from build123d import *

# Parameters (mm, degrees)
CYLINDER042_R          = 4
CYLINDER042_DEPTH      = 61
CYLINDER042_ROLL_ANGLE = 90
CYLINDER047_R          = 4
CYLINDER047_DEPTH      = 45
CYLINDER047_ROLL_ANGLE = 90
CYLINDER045_R          = 1.75
CYLINDER045_DEPTH      = 31
CYLINDER045_ROLL_ANGLE = 90
CYLINDER046_R          = 4
CYLINDER046_DEPTH      = 45
CYLINDER046_ROLL_ANGLE = 90
CYLINDER043_R          = 6
CYLINDER043_DEPTH      = 63
CYLINDER043_ROLL_ANGLE = 90
BOX038_W               = 8
BOX038_H               = 58
BOX038_DEPTH           = 11
CYLINDER044_R          = 1.75
CYLINDER044_DEPTH      = 23
CYLINDER044_ROLL_ANGLE = 90
BOX040_W               = 81
BOX040_H               = 81
BOX040_DEPTH           = 6
FILLET018008_R         = 5
BOX039_W               = 76
BOX039_H               = 76
BOX039_DEPTH           = 66
FILLET018007_R         = 3


with BuildPart() as cylinder064:
    # Cylinder042 → Cylinder042 (new body)
    with BuildSketch(Plane.XY):
        Circle(CYLINDER042_R)
    extrude(amount=CYLINDER042_DEPTH)


with BuildPart() as cylinder064_1:
    # Cylinder042 roll: moved
    add(cylinder064.part.rotate(Axis((0, 0, 0), (1, 0, 0)), CYLINDER042_ROLL_ANGLE))


with BuildPart() as cylinder064_2:
    # Cylinder042 placement: moved
    add(cylinder064_1.part.moved(Location((-5, 124, 89.6))))


with BuildPart() as cylinder069:
    # Cylinder047 → Cylinder047 (new body)
    with BuildSketch(Plane.XY):
        Circle(CYLINDER047_R)
    extrude(amount=CYLINDER047_DEPTH)


with BuildPart() as cylinder069_1:
    # Cylinder047 roll: moved
    add(cylinder069.part.rotate(Axis((0, 0, 0), (1, 0, 0)), CYLINDER047_ROLL_ANGLE))


with BuildPart() as cylinder069_2:
    # Cylinder047 placement: moved
    add(cylinder069_1.part.moved(Location((-8.5, 124, 71.5))))


with BuildPart() as cylinder067:
    # Cylinder045 → Cylinder045 (new body)
    with BuildSketch(Plane.XY):
        Circle(CYLINDER045_R)
    extrude(amount=CYLINDER045_DEPTH)


with BuildPart() as cylinder067_1:
    # Cylinder045 roll: moved
    add(cylinder067.part.rotate(Axis((0, 0, 0), (1, 0, 0)), CYLINDER045_ROLL_ANGLE))


with BuildPart() as cylinder067_2:
    # Cylinder045 placement: moved
    add(cylinder067_1.part.moved(Location((-8.5, 94, 71.5))))


with BuildPart() as cylinder068:
    # Cylinder046 → Cylinder046 (new body)
    with BuildSketch(Plane.XY):
        Circle(CYLINDER046_R)
    extrude(amount=CYLINDER046_DEPTH)


with BuildPart() as cylinder068_1:
    # Cylinder046 roll: moved
    add(cylinder068.part.rotate(Axis((0, 0, 0), (1, 0, 0)), CYLINDER046_ROLL_ANGLE))


with BuildPart() as cylinder068_2:
    # Cylinder046 placement: moved
    add(cylinder068_1.part.moved(Location((-8.5, -7, 71.5))))


with BuildPart() as cylinder065:
    # Cylinder043 → Cylinder043 (new body)
    with BuildSketch(Plane.XY):
        Circle(CYLINDER043_R)
    extrude(amount=CYLINDER043_DEPTH)


with BuildPart() as cylinder065_1:
    # Cylinder043 roll: moved
    add(cylinder065.part.rotate(Axis((0, 0, 0), (1, 0, 0)), CYLINDER043_ROLL_ANGLE))


with BuildPart() as cylinder065_2:
    # Cylinder043 placement: moved
    add(cylinder065_1.part.moved(Location((-3, 11, 83.5))))


with BuildPart() as cube037:
    # Box038 → Box038 (new body)
    with BuildSketch(Plane(origin=(-11.5, -52, 95), x_dir=(1, 0, 0), z_dir=(0, 0, 1))):
        with Locations((4, 29)):
            Rectangle(BOX038_W, BOX038_H)
    extrude(amount=BOX038_DEPTH)


with BuildPart() as cylinder066:
    # Cylinder044 → Cylinder044 (new body)
    with BuildSketch(Plane.XY):
        Circle(CYLINDER044_R)
    extrude(amount=CYLINDER044_DEPTH)


with BuildPart() as cylinder066_1:
    # Cylinder044 roll: moved
    add(cylinder066.part.rotate(Axis((0, 0, 0), (1, 0, 0)), CYLINDER044_ROLL_ANGLE))


with BuildPart() as cylinder066_2:
    # Cylinder044 placement: moved
    add(cylinder066_1.part.moved(Location((-8.5, 1, 71.5))))


with BuildPart() as fillet018008:
    # Box040 → Box040 (new body)
    with BuildSketch(Plane(origin=(-23.5, -4.5, 63), x_dir=(1, 0, 0), z_dir=(0, 0, 1))):
        with Locations((40.5, 40.5)):
            Rectangle(BOX040_W, BOX040_H)
    extrude(amount=BOX040_DEPTH)

    # Fillet018008
    fillet018008_edges = [fillet018008.edges().sort_by_distance(p)[0] for p in [
        (-23.5, -4.5, 66),
        (-23.5, 76.5, 66),
        (57.5, -4.5, 66),
        (57.5, 76.5, 66),
    ]]
    fillet(fillet018008_edges, radius=FILLET018008_R)


with BuildPart() as fillet018008_1:
    # Fillet018008 placement: moved
    add(fillet018008.part.moved(Location((0, 0, -1))))


with BuildPart() as corte_positivo:
    # Box039 → Box039 (new body)
    with BuildSketch(Plane(origin=(-21, -2, 63), x_dir=(1, 0, 0), z_dir=(0, 0, 1))):
        with Locations((38, 38)):
            Rectangle(BOX039_W, BOX039_H)
    extrude(amount=BOX039_DEPTH)

    # Fillet018007
    fillet018007_edges = [corte_positivo.edges().sort_by_distance(p)[0] for p in [
        (-21, -2, 96),
        (-21, 36, 129),
        (-21, 74, 96),
        (55, -2, 96),
        (55, 36, 129),
        (55, 74, 96),
        (17, -2, 129),
        (17, 74, 129),
    ]]
    fillet(fillet018007_edges, radius=FILLET018007_R)

    # Fusion033: union Fillet018008
    add(fillet018008_1.part)

    # Fusion034: union Cylinder064, Cylinder069, Cylinder067, Cylinder068, Cylinder065, Cube037, Cylinder066
    add(cylinder064_2.part)
    add(cylinder069_2.part)
    add(cylinder067_2.part)
    add(cylinder068_2.part)
    add(cylinder065_2.part)
    add(cube037.part)
    add(cylinder066_2.part)


solid = corte_positivo.part
The listing builds one solid part. Answer for the finished solid, in the listing's coordinates (mm). A direction names the side the tool comes from. Coordinates: 2 decimals unless noted, no trailing zeros. Write each loop counter-clockwise with the first axis right and the second up, starting at its lowest first coordinate (ties: lowest second). Pieces come first, ordered by that corner, then holes. Notation, with made-up numbers: (32.5, 4) - (61.5, 4) arc R12 ccw to (61.5, 15) - close; hole circle Ø11 at (-14.5, 85.5). An arc over 180 degrees is marked (long way). Put each result on its own line as item: value.
1. Flat-ended cylindrical pins translate along their axes: pin 1 Ø4 at (x, z) = (14, 80.5) entering from +Y; pin 2 Ø3.5 at (y, z) = (-21.5, 101) entering from +X; pin 3 Ø6 at (x, z) = (11.5, 100) entering from -Y. Find the tip coordinate at first contact, or state that the pin passes through.
Answer sheet:
pin 1: stops at y = 74
pin 2: stops at x = -3.5
pin 3: stops at y = -2
2. The part is cut by section C-C on x = 37. Give the vertices of the cut face in (y, z), plus the area to 3 significant figures.
Answer sheet:
outline: (-4.5, 62) - (76.5, 62) - (76.5, 68) - (74, 68) - (74, 126) arc R3 ccw to (71, 129) - (1, 129) arc R3 ccw to (-2, 126) - (-2, 68) - (-4.5, 68) - close
area: 5,120 mm^2
3. Determine the mould class of faces 1 (the face through (-9.367, 101.815, 67.595)), 2 (the face through (56, -3.07, 65.04)), 3 (the face through (-7.67, -7, 69.78)) for opening direction Y: pulls with the +Y half, pulls with the -Y half, needs draft (parallel to the pull), parting line crosses it, or undercut.
Answer sheet:
face 1: needs draft
face 2: pulls with the -Y half
face 3: undercut
4. Find the intervals of material crossed by line 1 along Z through (x, y) = (-8, -12); line 2 along X through (y, z) = (27.5, 125); line 3 along Z through (x, y) = (-7, -7.5), in increasing order. Write a range as from..to.
Answer sheet:
line 1: z = 67.53..75.47, 80.18..86.82, 95..106
line 2: x = -21..55
line 3: z = 67.79..75.21, 79.03..87.97, 95..106
5. A tool of negligible diameter and unlimited length cuts with its end or side. For faces 4 (the face through (-8.88, 76.54, 69.79)), 5 (the face through (55, 36, 97)), 6 (the face through (-8, -27, 95)), 7 (the face through (-3.5, -27, 100)), from which of +Z, -Z, +X, -X, +Y, -Y can it reach the whole face along a straight path? Write none if from no direction.
Answer sheet:
face 4: none
face 5: +Z, +X, +Y, -Y
face 6: +X, -X, -Y
face 7: +Z, +X, -Y
6. The part is cut by section B-B on z = 71.5. Give the vertices of the cut face in (x, y).
Answer sheet:
outline: (-21, 1) arc R3 ccw to (-18, -2) - (-10.25, -2) - (-10.25, -7) - (-12.5, -7) - (-12.5, -52) - (-4.5, -52) - (-4.5, -7) - (-6.75, -7) - (-6.75, -2) - (52, -2) arc R3 ccw to (55, 1) - (55, 71) arc R3 ccw to (52, 74) - (-6.75, 74) - (-6.75, 79) - (-4.5, 79) - (-4.5, 124) - (-12.5, 124) - (-12.5, 79) - (-10.25, 79) - (-10.25, 74) - (-18, 74) arc R3 ccw to (-21, 71) - close
7. The part is cut by section A-A on y = -36. Give the vertices of the cut face in (x, z).
Answer sheet:
outline: circle Ø8 at (-8.5, 71.5); (-11.5, 95) - (-3.5, 95) - (-3.5, 106) - (-11.5, 106) - close; circle Ø12 at (-3, 83.5)
8. The part is cut by section D-D on y = 21. Give the vertices of the cut face in (x, z), plus the area to 3 significant figures.
Answer sheet:
outline: (-23.5, 62) - (57.5, 62) - (57.5, 68) - (55, 68) - (55, 126) arc R3 ccw to (52, 129) - (-18, 129) arc R3 ccw to (-21, 126) - (-21, 68) - (-23.5, 68) - close
area: 5,120 mm^2
